Part model, mm, in its own coordinate system. Round coordinates to 2 decimals unless told otherwise and drop trailing zeros. Write each loop counter-clockwise with the first axis right and the second up, starting at its lowest first coordinate (ties: lowest second). Pieces come first, ordered by that corner, then holes.
```python
from build123d import *

# Parameters (mm, degrees)
SKETCH1_W                        = 520
SKETCH1_H                        = 446
BOSS_EXTRUDE1_DEPTH              = 10
SKETCH4_W                        = 480
SKETCH4_H                        = 50
CUT_EXTRUDE1_DEPTH               = 10
FILLET1_R                        = 5
CHAMFER1_SIZE                    = 2.5
CBORE_FOR_M4_SHCS1_D             = 4.5
CBORE_FOR_M4_SHCS1_DEPTH         = 12
CBORE_FOR_M4_SHCS1_CBORE_D       = 8
CBORE_FOR_M4_SHCS1_CBORE_DEPTH   = 4
CBORE_FOR_M4_SHCS1_TIP           = 1.351936393
M4X0_7_TAPPED_HOLE1_D            = 3.3
CBORE_FOR_M2_5_SHCS1_D           = 2.9
CBORE_FOR_M2_5_SHCS1_CBORE_D     = 5.5
CBORE_FOR_M2_5_SHCS1_CBORE_DEPTH = 2.5
M2_5X0_45_TAPPED_HOLE1_D         = 2.05


with BuildPart() as part:
    # Sketch1 → Boss-Extrude1 (new body)
    with BuildSketch(Plane(origin=(0, 0, 0), x_dir=(1, 0, 0), z_dir=(0, 1, 0))):
        with Locations((260, 223)):
            Rectangle(SKETCH1_W, SKETCH1_H)
    extrude(amount=BOSS_EXTRUDE1_DEPTH)

    # Sketch4 → Cut-Extrude1 (cut)
    with BuildSketch(Plane(origin=(0, 10, 0), x_dir=(1, 0, 0), z_dir=(0, 1, 0))):
        with Locations((260, 391)):
            Rectangle(SKETCH4_W, SKETCH4_H)
    extrude(amount=-CUT_EXTRUDE1_DEPTH, mode=Mode.SUBTRACT)

    # Fillet1
    fillet1_edges = [part.edges().sort_by_distance(p)[0] for p in [
        (500, 5, -416),
        (500, 5, -366),
        (20, 5, -366),
        (20, 5, -416),
    ]]
    fillet(fillet1_edges, radius=FILLET1_R)

    # Chamfer1
    chamfer1_edges = [part.edges().sort_by_distance(p)[0] for p in [
        (500, 10, -391),
        (500, 0, -391),
        (260, 10, -366),
        (260, 0, -366),
        (20, 10, -391),
        (20, 0, -391),
        (260, 10, -416),
        (260, 0, -416),
        (498.535533906, 10, -367.464466094),
        (498.535533906, 0, -367.464466094),
        (21.464466094, 10, -414.535533906),
        (21.464466094, 0, -414.535533906),
        (498.535533906, 10, -414.535533906),
        (498.535533906, 0, -414.535533906),
        (21.464466094, 10, -367.464466094),
        (21.464466094, 0, -367.464466094),
    ]]
    chamfer(chamfer1_edges, length=CHAMFER1_SIZE)

    # CBORE for M4 SHCS1
    with Locations(Plane(origin=(0, 10, 0), x_dir=(1, 0, 0), z_dir=(0, 1, 0))):
        with Locations((5, 373), (5, 223), (5, 73), (70, 5), (260, 5), (450, 5), (515, 73), (515, 223), (515, 373), (450, 441), (260, 441), (70, 441)):
            CounterBoreHole(CBORE_FOR_M4_SHCS1_D / 2, CBORE_FOR_M4_SHCS1_CBORE_D / 2, CBORE_FOR_M4_SHCS1_CBORE_DEPTH, depth=CBORE_FOR_M4_SHCS1_DEPTH)
            with Locations((0, 0, -(CBORE_FOR_M4_SHCS1_DEPTH + CBORE_FOR_M4_SHCS1_TIP / 2))):  # 118° drill point
                Cone(0, CBORE_FOR_M4_SHCS1_D / 2, CBORE_FOR_M4_SHCS1_TIP, mode=Mode.SUBTRACT)

    # M4x0.7 Tapped Hole1 (through all)
    with Locations(Plane(origin=(0, 10, 0), x_dir=(1, 0, 0), z_dir=(0, 1, 0))):
        with Locations((15, 431), (505, 431), (15, 15), (505, 15)):
            Hole(M4X0_7_TAPPED_HOLE1_D / 2)

    # CBORE for M2.5 SHCS1 (through all)
    with Locations(Plane(origin=(0, 10, 0), x_dir=(1, 0, 0), z_dir=(0, 1, 0))):
        with Locations((30, 33), (225, 33), (420, 33), (420, 323), (225, 323), (30, 323)):
            CounterBoreHole(CBORE_FOR_M2_5_SHCS1_D / 2, CBORE_FOR_M2_5_SHCS1_CBORE_D / 2, CBORE_FOR_M2_5_SHCS1_CBORE_DEPTH)

    # M2.5x0.45 Tapped Hole1 (through all)
    with Locations(Plane(origin=(0, 10, 0), x_dir=(1, 0, 0), z_dir=(0, 1, 0))):
        with Locations((54.288, 177.08759), (225.088, 177.08759)):
            Hole(M2_5X0_45_TAPPED_HOLE1_D / 2)


solid = part.part
```
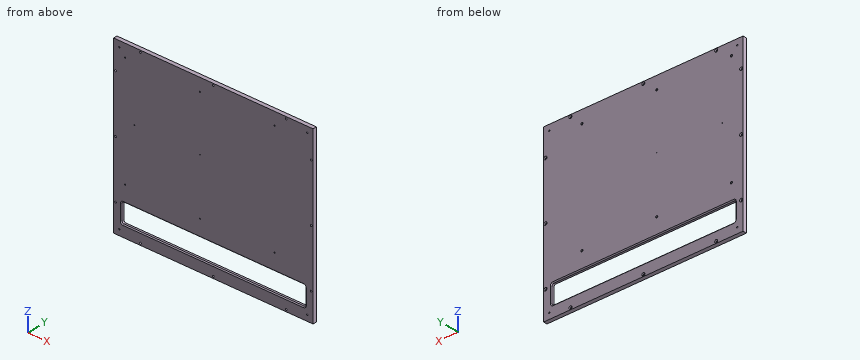
Q1. Wall check: L1, parallel to X at y = 9.15, z = -223; L2, parallel to X at y = 3.5, z = -431; L3, parallel to Z at x = 5, y = 4. Give the ranges that are in metal, low to high.
Values follow:
L1: x = 0 to 1, 9 to 511, 519 to 520
L2: x = 0 to 13.35, 16.65 to 503.35, 506.65 to 520
L3: z = -446 to -375.25, -370.75 to -225.25, -220.75 to -75.25, -70.75 to 0
Q2. Drop flat-ended pins along their axis: pin 1 (7 mm diameter, centred on x = 260, z = -441, fed in from +Y); pin 2 (3 mm diameter, centred on x = 98.5, z = -281.5, fed in from -Y); pin 3 (2.5 mm diameter, centred on x = 225, z = -323, fed in from +Y); pin 4 (5 mm diameter, centred on x = 420, z = -33, fed in from +Y). Give the stop position or say it passes through.
Values follow:
pin 1: stops at y = 6
pin 2: stops at y = 0
pin 3: passes through
pin 4: stops at y = 7.5
Q3. Cut at A-A on x = 137. Write the cut outline in (y, z).
Values follow:
outline: (0, -446) - (10, -446) - (10, -418.5) - (7.5, -416) - (2.5, -416) - (0, -418.5) - close; (0, -363.5) - (2.5, -366) - (7.5, -366) - (10, -363.5) - (10, 0) - (0, 0) - close
